```python
from build123d import *

# Parameters (mm, degrees)
SKETCH1_W           = 86.36
SKETCH1_H           = 95.25
SKETCH1_W_2         = 71.12
SKETCH1_H_2         = 80.01
BOSS_EXTRUDE1_DEPTH = 12.7
FILLET1_R           = 3.175


with BuildPart() as part:
    # Sketch1 → Boss-Extrude1 (new body)
    with BuildSketch(Plane.XY):
        with Locations((-43.18, 47.625)):
            Rectangle(SKETCH1_W, SKETCH1_H)
        with Locations((-43.18, 47.625)):
            Rectangle(SKETCH1_W_2, SKETCH1_H_2, mode=Mode.SUBTRACT)
    extrude(amount=BOSS_EXTRUDE1_DEPTH)

    # Fillet1
    fillet1_edges = [part.edges().sort_by_distance(p)[0] for p in [
        (-86.36, 47.625, 12.7),
        (-43.18, 0, 12.7),
        (0, 47.625, 12.7),
        (-43.18, 0, 0),
        (-86.36, 47.625, 0),
        (-43.18, 95.25, 0),
        (0, 47.625, 0),
        (0, 0, 6.35),
        (-86.36, 0, 6.35),
        (-86.36, 95.25, 6.35),
        (0, 95.25, 6.35),
        (-43.18, 95.25, 12.7),
    ]]
    fillet(fillet1_edges, radius=FILLET1_R)


solid = part.part
```
CAD build for the part. Positions are in the model's coordinates, mm. A direction names the side the tool comes from. Give positions to 0.01 mm unless a question says otherwise; leave off trailing zeros. Loops run counter-clockwise (first coordinate to the right, second up) from the corner with the lowest first, then second, coordinate; pieces in that order, holes last. Notation, with made-up numbers: M 56,60.5 L 90,60.5 A34 cw 90,90.5 Z; hole C 74.25,26.25 d3. An arc over 180 degrees is marked long. Use one line per item in the form item = value.
Item 1: Slice it at C-C (x = -72). List the corners of the cut face in (y, z) (3 decimals), plus the area to 3 significant figures.
Determined:
outline = M 0,3.175 A3.175 ccw 3.175,0 L 7.62,0 L 7.62,12.7 L 3.175,12.7 A3.175 ccw 0,9.525 Z; M 87.63,0 L 92.075,0 A3.175 ccw 95.25,3.175 L 95.25,9.525 A3.175 ccw 92.075,12.7 L 87.63,12.7 Z
area = 185 mm2
Item 2: Two-plate mould, pull along Y, no slides. Class faces 1 (the face through (-42.62, 94.34, 0.95)), 2 (the face through (-44, 0, 6)), 3 (the face through (-44, 87.63, 6)): pulls with the +Y half, pulls with the -Y half, needs draft (parallel to the pull), parting line crosses it, or undercut.
Determined:
face_1 = pulls with the +Y half
face_2 = pulls with the -Y half
face_3 = undercut
Item 3: Which spindle directions (+Z, -Z, +X, -X, +Y, -Y) get a long thin tool onto all of the face, cutting with end or side? Do faces 4 (the face through (-44, 7.62, 6)), 5 (the face through (-85.5, 48.2, 11.7)). Say none if no direction does.
Determined:
face_4 = +Z, -Z
face_5 = +Z, -X, +Y, -Y
Item 4: Drill centre lines: probe 1 along Y at (x, z) = (-39, 5); probe 2 along X at (y, z) = (12.5, 6.75); probe 3 along Y at (x, z) = (-9, 2). Where is each one in solid material? Low to high. Write a range as from..to.
Determined:
probe_1 = 0..7.62, 87.63..95.25
probe_2 = -86.36..-78.74, -7.62..0
probe_3 = 0.23..7.62, 87.63..95.02
Item 5: Flat gauge pin, fed straight in: pin 1 (5 mm diameter, centred on x = -34, z = 10, fed in from +Y). Where does the tip first touch, or does it go through?
Determined:
pin_1 = 95.25
Item 6: Slice it at B-B (z = 6). List the corners of the cut face in (x, y) (3 decimals).
Determined:
outline = M -86.36,3.175 A3.175 ccw -83.185,0 L -3.175,0 A3.175 ccw 0,3.175 L 0,92.075 A3.175 ccw -3.175,95.25 L -83.185,95.25 A3.175 ccw -86.36,92.075 Z; hole M -78.74,7.62 L -7.62,7.62 L -7.62,87.63 L -78.74,87.63 Z
Item 7: Slice it at A-A (y = 60.5). List the corners of the cut face in (x, z) (3 decimals).
Determined:
outline = M -86.36,3.175 A3.175 ccw -83.185,0 L -78.74,0 L -78.74,12.7 L -83.185,12.7 A3.175 ccw -86.36,9.525 Z; M -7.62,0 L -3.175,0 A3.175 ccw 0,3.175 L 0,9.525 A3.175 ccw -3.175,12.7 L -7.62,12.7 Z
